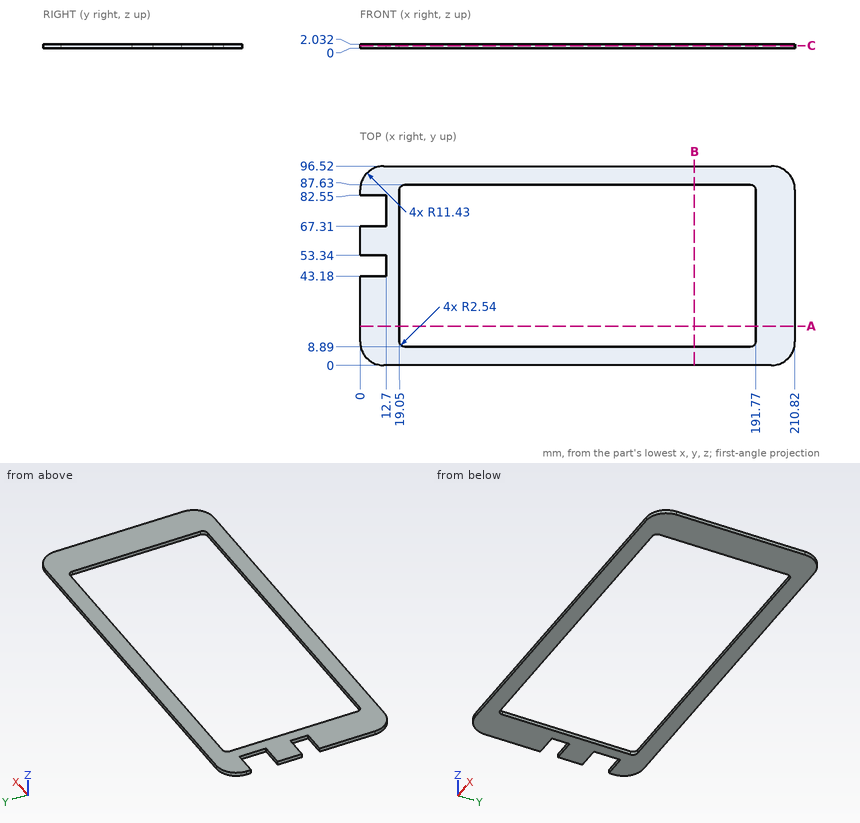
Geometry: see drawing. Coordinates: mm, zero at the bounding-box minimum. Coordinates: 2 decimals unless noted, no trailing zeros. Order: outer loops, then holes, each group sorted by start corner. A loop starts at its lowest first (then second) coordinate and runs counter-clockwise, first axis right, second up. Notation, with made-up numbers: (51, -9) - (110, -9) arc R11 ccw to (110, 1) - close; hole circle Ø7 at (41.5, 17.5). An arc over 180 degrees is marked (long way). Return JSON: item names as keys, results as strings.
Q1. Cut plane C-C (z = 1.25). Return loops of the section in (x, y).
The answers:
{"outline": "(0, 11.43) arc R11.43 ccw to (11.43, 0) - (199.39, 0) arc R11.43 ccw to (210.82, 11.43) - (210.82, 85.09) arc R11.43 ccw to (199.39, 96.52) - (11.43, 96.52) arc R11.43 ccw to (0, 85.09) - (0, 82.55) - (12.7, 82.55) - (12.7, 67.31) - (0, 67.31) - (0, 53.34) - (12.7, 53.34) - (12.7, 43.18) - (0, 43.18) - close; hole (19.05, 11.43) arc R2.54 ccw to (21.59, 8.89) - (189.23, 8.89) arc R2.54 ccw to (191.77, 11.43) - (191.77, 85.09) arc R2.54 ccw to (189.23, 87.63) - (21.59, 87.63) arc R2.54 ccw to (19.05, 85.09) - close"}
Q2. Cut plane B-B (x = 162). Return loops of the section in (y, z).
The answers:
{"outline": "(0, 0) - (8.89, 0) - (8.89, 2.03) - (0, 2.03) - close; (87.63, 0) - (96.52, 0) - (96.52, 2.03) - (87.63, 2.03) - close"}
Q3. Cut plane A-A (y = 19). Return loops of the section in (x, z).
The answers:
{"outline": "(0, 0) - (19.05, 0) - (19.05, 2.03) - (0, 2.03) - close; (191.77, 0) - (210.82, 0) - (210.82, 2.03) - (191.77, 2.03) - close"}
Q4. First-contact query: pin 1 (1 mm diameter, centred on x = 3.5, z = 0.5, fed in from +Y); pin 2 (0.6 mm diameter, centred on x = 7, z = 1, fed in from +Y). Flat tips, straight axial feed; report the tip coordinate or a pass-through.
The answers:
{"pin 1": "stops at y = 93.78", "pin 2": "stops at y = 95.75"}
Q5. Ray query, probe 1 along Y at (x, z) = (117, 1.8); probe 2 along X at (y, z) = (49, 1.85); probe 3 along X at (y, z) = (36, 0.25). Return the intervals inside material, ascending.
The answers:
{"probe 1": "y = 0 to 8.89, 87.63 to 96.52", "probe 2": "x = 12.7 to 19.05, 191.77 to 210.82", "probe 3": "x = 0 to 19.05, 191.77 to 210.82"}
